The model under review builds one solid part; all positions refer to its coordinate system, in mm. Face numbers are marked on the shaded views. Coordinates: 2 decimals unless noted, no trailing zeros. Loops run counter-clockwise (first coordinate to the right, second up) from the corner with the lowest first, then second, coordinate; pieces in that order, holes last. Notation, with made-up numbers: (26, -36) - (80, -36) arc R13 cw to (80, -20) - close; hole circle Ø2 at (-1.75, -25.75). An arc over 180 degrees is marked (long way). Use a Markdown table: item, result. Add a question column.
1) Add section C-C, the plane y = 13.25. Give the boundary of the cut face in (x, z).
2) The part is to be moulded in two halves that separate along Z. For the marked faces 1, 2, 3 and 4, say which applies: pulls with the +Z half, pulls with the -Z half, needs draft (parallel to the pull), parting line crosses it, or undercut.
3) Add section B-B, the plane z = 8. Give the boundary of the cut face in (x, y).
4) Clearance check with flat-ended pins moving along their axes: pin 1 (2 mm diameter, centred on x = -3, z = -8.5, fed in from -Y); pin 2 (3 mm diameter, centred on x = 0, z = -8, fed in from -Y); pin 3 (2 mm diameter, centred on y = 7, z = 5.5, fed in from +X); pin 4 (3 mm diameter, centred on x = -1.5, z = 7.5, fed in from +Y). State where each tip first meets the part, or that it passes through.
5) Add section A-A, the plane x = 0. Give the boundary of the cut face in (y, z).
6) To check wall thickness, follow L1, parallel to X at y = 11.5, z = 0; L2, parallel to X at y = 12.1, z = -8; L3, parallel to Y at x = -3.5, z = 8. State the ranges of each line that lie inside material, in increasing order. Write a range as [from, to].
7) Add section D-D, the plane y = 6.5. Give the boundary of the cut face in (x, z), and give its area (3 significant figures).
```python
from build123d import *

# Parameters (mm, degrees)
SKETCH1_R           = 5.1
BOSS_EXTRUDE1_DEPTH = 15
SKETCH2_R           = 1.75
BOSS_EXTRUDE2_DEPTH = 3.5
SKETCH3_R           = 3.35
CUT_EXTRUDE1_DEPTH  = 20.287560758


with BuildPart() as part:
    # Sketch1 → Boss-Extrude1 (new body)
    with BuildSketch(Plane(origin=(0, 0, 0), x_dir=(1, 0, 0), z_dir=(0, 1, 0))):
        with Locations(Location((0, 0, 0), (0, 0, 270))):
            Circle(SKETCH1_R)
    extrude(amount=BOSS_EXTRUDE1_DEPTH)

    # Sketch2 → Boss-Extrude2 (add)
    with BuildSketch(Plane(origin=(0, 13.5, 0), x_dir=(1, 0, 0), z_dir=(0, 1, 0))):
        with BuildLine():
            Line((-5.1, 9.746281342), (-5.1, -9.746281342))
            ThreePointArc((-5.1, -9.746281342), (0, -11), (5.1, -9.746281342))
            Line((5.1, -9.746281342), (5.1, 9.746281342))
            ThreePointArc((5.1, 9.746281342), (0, 11), (-5.1, 9.746281342))
        make_face()
        with Locations(Location((0, 8, 0), (0, 0, 270))):
            Circle(SKETCH2_R, mode=Mode.SUBTRACT)
        with Locations(Location((0, -8, 0), (0, 0, 270))):
            Circle(SKETCH2_R, mode=Mode.SUBTRACT)
    extrude(amount=-BOSS_EXTRUDE2_DEPTH)

    # Sketch3 → Cut-Extrude1 (cut, through all)
    with BuildSketch(Plane(origin=(0, 15, 0), x_dir=(1, 0, 0), z_dir=(0, 1, 0))):
        with Locations(Location((0, 0, 0), (0, 0, 270))):
            Circle(SKETCH3_R)
    extrude(amount=-CUT_EXTRUDE1_DEPTH, mode=Mode.SUBTRACT)


solid = part.part
```
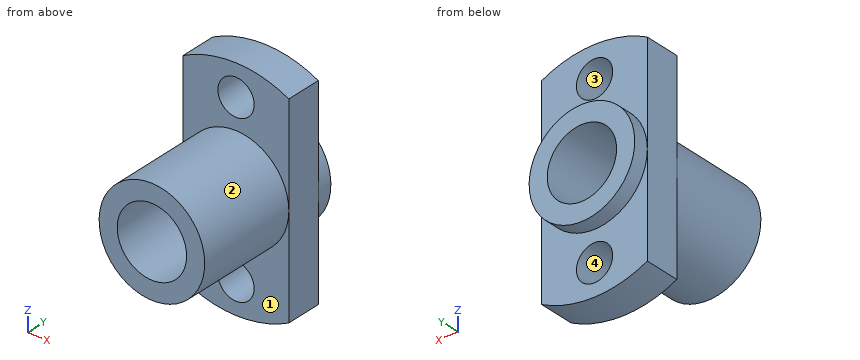
From the geometry:
| question | item | result |
|---|---|---|
| 1 | outline | (-5.1, -9.75) arc R11 ccw to (5.1, -9.75) - (5.1, 9.75) arc R11 ccw to (-5.1, 9.75) - close; hole circle Ø6.7 at (0, 0); hole circle Ø3.5 at (0, -8); hole circle Ø3.5 at (0, 8) |
| 2 | face 1 | needs draft |
| 2 | face 2 | parting line crosses it |
| 2 | face 3 | undercut |
| 2 | face 4 | undercut |
| 3 | outline | (-5.1, 10) - (-1.75, 10) - (-1.75, 13.5) - (-5.1, 13.5) - close; (1.75, 10) - (5.1, 10) - (5.1, 13.5) - (1.75, 13.5) - close |
| 4 | pin 1 | stops at y = 10 |
| 4 | pin 2 | passes through |
| 4 | pin 3 | stops at x = 2.4 |
| 4 | pin 4 | stops at y = 13.5 |
| 5 | outline | (0, -5.1) - (10, -5.1) - (10, -6.25) - (13.5, -6.25) - (13.5, -5.1) - (15, -5.1) - (15, -3.35) - (0, -3.35) - close; (0, 3.35) - (15, 3.35) - (15, 5.1) - (13.5, 5.1) - (13.5, 6.25) - (10, 6.25) - (10, 5.1) - (0, 5.1) - close; (10, -11) - (13.5, -11) - (13.5, -9.75) - (10, -9.75) - close; (10, 9.75) - (13.5, 9.75) - (13.5, 11) - (10, 11) - close |
| 6 | L1 | x = [-5.1, -3.35], [3.35, 5.1] |
| 6 | L2 | x = [-5.1, -1.75], [1.75, 5.1] |
| 6 | L3 | y = [10, 13.5] |
| 7 | outline | circle Ø10.2 at (0, 0); hole circle Ø6.7 at (0, 0) |
| 7 | area | 46.5 mm^2 |
